from build123d import *

# Parameters (mm, degrees)
SKETCH1_R           = 2
BOSS_EXTRUDE1_DEPTH = 8
SKETCH2_W           = 4
SKETCH2_H           = 2
SKETCH2_H_2         = 3
CUT_EXTRUDE1_DEPTH  = 8


with BuildPart() as part:
    # Sketch1 → Boss-Extrude1 (new body)
    with BuildSketch(Plane(origin=(0, 0, 0), x_dir=(1, 0, 0), z_dir=(0, 1, 0))):
        with BuildLine():
            Line((170, 4), (0, 4))
            ThreePointArc((0, 4), (-4, 0), (0, -4))
            Line((0, -4), (170, -4))
            ThreePointArc((170, -4), (174, 0), (170, 4))
        make_face()
        with Locations(Location((0, 0, 0), (0, 0, 270))):
            Circle(SKETCH1_R, mode=Mode.SUBTRACT)
        with Locations(Location((170, 0, 0), (0, 0, 270))):
            Circle(SKETCH1_R, mode=Mode.SUBTRACT)
    extrude(amount=BOSS_EXTRUDE1_DEPTH)

    # Sketch2 → Cut-Extrude1 (cut)
    with BuildSketch(Plane.XY.offset(4)):
        Polygon((22.660254038, 5), (0, 5), (0, 3), (19.196152423, 3), align=None)
        with Locations((-2, 4)):
            Rectangle(SKETCH2_W, SKETCH2_H)
        with Locations((-2, 6.5)):
            Rectangle(SKETCH2_W, SKETCH2_H_2)
        Polygon((0, 8), (0, 5), (22.660254038, 5), (27.856406461, 8), align=None)
        Polygon((170, 3), (25.196152423, 3), (20, 0), (170, 0), align=None)
        Polygon((170, 5), (28.660254038, 5), (25.196152423, 3), (170, 3), align=None)
        with Locations((172, 4)):
            Rectangle(SKETCH2_W, SKETCH2_H)
        with Locations((172, 1.5)):
            Rectangle(SKETCH2_W, SKETCH2_H_2)
    extrude(amount=-CUT_EXTRUDE1_DEPTH, mode=Mode.SUBTRACT)


solid = part.part
Source: CAD feature listing. Evaluate the final solid. Frame: model axes, mm. A direction names the side the tool comes from. Coordinates: 2 decimals unless noted, no trailing zeros. Loops run counter-clockwise (first coordinate to the right, second up) from the corner with the lowest first, then second, coordinate; pieces in that order, holes last. Notation, with made-up numbers: (-2.5, 69.5) -> (39.5, 69.5) arc R16 ccw to (39.5, 80.5) -> close; hole circle Ø8 at (52.5, 39). An arc over 180 degrees is marked (long way). Answer in a Markdown table with one row per item. Add a question column.
Q1. Section A-A on z = 0. Return the cut outline in (x, y).
Q2. Section B-B on x = 92. Return the cut outline in (y, z), and give its area (3 significant figures).
Q3. Contact query for flat-ended pins moving along their axis: pin 1 Ø1.5 at (y, z) = (6, 1.5) entering from +X; pin 2 Ø4 at (x, z) = (27, -3) entering from +Y; pin 3 Ø4 at (x, z) = (52.5, -2) entering from -Y. Output: stop coordinate, or through.
Q4. Pull-direction query (Z, two-part tool) for faces 1 (the face through (174, 6, 0)), 2 (the face through (100, 8, 0)), 3 (the face through (168.226, 6.479, 0.923)), 4 (the face through (85, 6, 4)); classes: pulls with the +Z half, pulls with the -Z half, needs draft (parallel to the pull), parting line crosses it, or undercut.
Q5. Reachability of faces 5 (the face through (102, 5, 0)), 6 (the face through (-2, 1, 0)), 7 (the face through (7, 3, 0)) from +Z, -Z, +X, -X, +Y, -Y: full face, straight path, thin tool, end or side. Return the list, or none.
Q6. Ray query, line 1 along Z through (x, y) = (170, 6.6); line 2 along Y through (x, z) = (151.5, 1.5); line 3 along X through (y, z) = (5.95, 0). Return the intervals inside material, ascending.
Computed values:
| question | item | result |
|---|---|---|
| 1 | outline | (-4, 0) -> (-2, 0) -> (-2, 3) -> (-4, 3) -> close; (2, 0) -> (20, 0) -> (28.66, 5) -> (168, 5) -> (168, 8) -> (27.86, 8) -> (19.2, 3) -> (2, 3) -> close; (172, 5) -> (174, 5) -> (174, 8) -> (172, 8) -> close |
| 2 | outline | (5, -4) -> (8, -4) -> (8, 4) -> (5, 4) -> close |
| 2 | area | 24.0 mm^2 |
| 3 | pin 1 | stops at x = 173.93 |
| 3 | pin 2 | stops at y = 8 |
| 3 | pin 3 | stops at y = 5 |
| 4 | face 1 | parting line crosses it |
| 4 | face 2 | needs draft |
| 4 | face 3 | undercut |
| 4 | face 4 | pulls with the +Z half |
| 5 | face 5 | +Z, -Z, +X, -Y |
| 5 | face 6 | +Y, -Y |
| 5 | face 7 | +Z, -Z, -X, +Y |
| 6 | line 1 | z = -4 to -2, 2 to 4 |
| 6 | line 2 | y = 5 to 8 |
| 6 | line 3 | x = 24.31 to 168, 172 to 174 |
